Here's how the part is built. I have some questions about the finished solid (model axes, mm). A direction names the side the tool comes from. Give positions to 0.01 mm unless a question says otherwise; leave off trailing zeros. Write each loop counter-clockwise with the first axis right and the second up, starting at its lowest first coordinate (ties: lowest second). Pieces come first, ordered by that corner, then holes. Notation, with made-up numbers: (63, -31) -> (95, -31) arc R29 ccw to (95, 0) -> close; hole circle Ø5 at (76.5, -37). An arc over 180 degrees is marked (long way). Use one line per item in the form item = value.
```python
from build123d import *

# Parameters (mm, degrees)
F1_DEPTH = 25.4
F3_DEPTH = 25.4
F5_R     = 6.35


with BuildPart() as f1:
    # F0 (on Front) → F1 (new body)
    with BuildSketch(Plane.XZ):
        Polygon((-12.7, 0), (0, 0), (12.7, 0), (12.7, 38.1), (0, 38.1), (-12.7, 38.1), align=None)
    extrude(amount=F1_DEPTH)

    # F2 (on face) → F3 (join)
    with BuildSketch(Plane.XY.offset(38.1)):
        Polygon((5.715, -6.985), (0, -6.985), (0, -12.7), (0, -18.415), (5.715, -18.415), align=None)
        Polygon((0, -12.7), (0, -6.985), (-5.715, -6.985), (-5.715, -18.415), (0, -18.415), align=None)
    extrude(amount=F3_DEPTH)

    # F4: F1 across plane


with BuildPart() as f1_1:
    add(f1.part)
    add(f1.part.mirror(Plane.XY))

    # F5
    f5_edges = [f1_1.edges().sort_by_distance(p)[0] for p in [
        (12.7, 0, 0),
        (12.7, -25.4, 0),
        (-12.7, 0, 0),
        (-12.7, -25.4, 0),
    ]]
    fillet(f5_edges, radius=F5_R)


solid = f1_1.part
```
Q1. If I drill on line 1 along Z through (x, y) = (5.75, -1.25); line 2 along X through (y, z) = (-5.5, 17.5); line 3 along Y through (x, z) = (-7, 2), over which ranges is the centre line in solid material (lowest first)? Write a range as from..to.
Result set:
line_1 = -38.1..38.1
line_2 = -12.64..12.64
line_3 = -25.37..-0.03
Q2. I want a section at D-D, the plane z = 48.5. Write out the boundary of the cut face in (x, y) (3 decimals).
Result set:
outline = (-5.715, -18.415) -> (5.715, -18.415) -> (5.715, -6.985) -> (-5.715, -6.985) -> close
Q3. I want a section at A-A, the plane y = -11.25. Write out the boundary of the cut face in (x, z) (3 decimals).
Result set:
outline = (-12.7, -38.1) -> (-5.715, -38.1) -> (-5.715, -63.5) -> (5.715, -63.5) -> (5.715, -38.1) -> (12.7, -38.1) -> (12.7, 38.1) -> (5.715, 38.1) -> (5.715, 63.5) -> (-5.715, 63.5) -> (-5.715, 38.1) -> (-12.7, 38.1) -> close
Q4. I want a section at B-B, the plane z = -30. Write out the boundary of the cut face in (x, y).
Result set:
outline = (-12.7, -19.05) arc R6.35 ccw to (-6.35, -25.4) -> (6.35, -25.4) arc R6.35 ccw to (12.7, -19.05) -> (12.7, -6.35) arc R6.35 ccw to (6.35, 0) -> (-6.35, 0) arc R6.35 ccw to (-12.7, -6.35) -> close
Q5. I want a section at C-C, the plane x = 3.5. Write out the boundary of the cut face in (y, z) (3 decimals), and give its area (3 significant figures).
Result set:
outline = (-25.4, -38.1) -> (-18.415, -38.1) -> (-18.415, -63.5) -> (-6.985, -63.5) -> (-6.985, -38.1) -> (0, -38.1) -> (0, 38.1) -> (-6.985, 38.1) -> (-6.985, 63.5) -> (-18.415, 63.5) -> (-18.415, 38.1) -> (-25.4, 38.1) -> close
area = 2,520 mm2
Q6. Will these pins go through, and if not, where does the flat tip stop? pin 1 Ø9 at (y, z) = (-13.5, 49) entering from +X (3 decimals); pin 2 Ø9 at (y, z) = (-15, -49) entering from -X (3 decimals); pin 3 Ø12.5 at (x, z) = (0, 52) entering from +Y (3 decimals).
Result set:
pin_1 = 5.715
pin_2 = -5.715
pin_3 = -6.985
Q7. Which directions (+Z, -Z, +X, -X, +Y, -Y) give clear straight access to the entire face, cutting with the end or side of a thin tool? Please do faces 1 (the face through (5.715, -13, -51)), 2 (the face through (-5.715, -13, 51)), 3 (the face through (0, -18.415, -51)), 4 (the face through (5.715, -13, 51)).
Result set:
face_1 = -Z, +X, +Y, -Y
face_2 = +Z, -X, +Y, -Y
face_3 = -Z, +X, -X, -Y
face_4 = +Z, +X, +Y, -Y
